from build123d import *

# Parameters (mm, degrees)
SKETCH_1_W          = 85
SKETCH_1_H          = 40
EXTRUDE_1_DEPTH     = 30
SKETCH_2_W          = 60
SKETCH_2_H          = 10
CUT_EXTRUDE_2_DEPTH = 112.467484048
SKETCH_3_R          = 11
CUT_EXTRUDE_3_DEPTH = 99.615414617


with BuildPart() as part:
    # 草图1 → 凸台-拉伸1 (new, symmetric)
    with BuildSketch(Plane.XY):
        with Locations((-42.5, -20)):
            Rectangle(SKETCH_1_W, SKETCH_1_H)
    extrude(amount=EXTRUDE_1_DEPTH, both=True)

    # 草图2 → 切除-拉伸2 (cut, through all)
    with BuildSketch(Plane.XY.offset(30)):
        with Locations((-30, -35)):
            Rectangle(SKETCH_2_W, SKETCH_2_H)
    extrude(amount=-CUT_EXTRUDE_2_DEPTH, mode=Mode.SUBTRACT)

    # 草图3 → 切除-拉伸3 (cut, through all)
    with BuildSketch(Plane(origin=(0, 0, 0), x_dir=(1, 0, 0), z_dir=(0, 1, 0))):
        with Locations(Location((-30, 0, 0), (0, 0, 180))):
            Circle(SKETCH_3_R)
    extrude(amount=-CUT_EXTRUDE_3_DEPTH, mode=Mode.SUBTRACT)


solid = part.part
Source: CAD feature listing. Evaluate the final solid. Frame: model axes, mm. A direction names the side the tool comes from. Give positions to 0.01 mm unless a question says otherwise; leave off trailing zeros. Write each loop counter-clockwise with the first axis right and the second up, starting at its lowest first coordinate (ties: lowest second). Pieces come first, ordered by that corner, then holes. Notation, with made-up numbers: M 13,5.5 L 44,5.5 A5 cw 44,14.5 Z; hole C 36.5,-14 d5. An arc over 180 degrees is marked long. Return JSON: item names as keys, results as strings. Group by question number.
1) Set-up query: faces 1 (the face through (-85, -20, 0)), 2 (the face through (-60, -35, 0)). Return all of +Z, -Z, +X, -X, +Y, -Y with unobstructed straight access to the full face (end or side cutting, diameter ignored); none if empty.
2) Cut plane D-D, the plane z = 17. Output: boundary loops of the cut face in (x, y), then the cut area to 3 significant figures.
3) Draft query along Z for faces 3 (the face through (-40.492, -14.79, 3.304)), 4 (the face through (-73, -40, 0)), 5 (the face through (-43, -15, 30)). Return one class per face: released by +Z, released by -Z, zero draft, split by the parting line, or undercut.
4) Cut plane A-A, the plane z = 0. Output: boundary loops of the cut face in (x, y), then the cut area to 3 significant figures.
5) Ray query, L1, parallel to Z at x = -30.5, y = -26; L2, parallel to Y at x = -57, z = 0; L3, parallel to X at y = -35.5, z = -22. Return the intervals inside material, ascending.
6) First-contact query: pin 1 Ø3 at (y, z) = (-34, -6.5) entering from +X. Flat tip, straight axial feed; report the tip coordinate or a pass-through.
7) Cut plane C-C, the plane y = -14. Output: boundary loops of the cut face in (x, z), then the cut area to 3 significant figures.
8) Cut plane B-B, the plane x = -30. Output: boundary loops of the cut face in (y, z).
Data:
{
 "1": {"face 1": "+Z, -Z, -X, +Y, -Y", "face 2": "+Z, -Z, +X, -Y"},
 "2": {"outline": "M -85,-40 L -60,-40 L -60,-30 L 0,-30 L 0,0 L -85,0 Z", "area": "2,800 mm²"},
 "3": {"face 3": "undercut", "face 4": "zero draft", "face 5": "released by +Z"},
 "4": {"outline": "M -85,-40 L -60,-40 L -60,-30 L -41,-30 L -41,0 L -85,0 Z; M -19,-30 L 0,-30 L 0,0 L -19,0 Z", "area": "2,140 mm²"},
 "5": {"L1": "z = -30 to -10.99, 10.99 to 30", "L2": "y = -30 to 0", "L3": "x = -85 to -60"},
 "6": {"pin 1": "stops at x = -60"},
 "7": {"outline": "M -85,-30 L 0,-30 L 0,30 L -85,30 Z; hole C -30,0 d22", "area": "4,720 mm²"},
 "8": {"outline": "M -30,-30 L 0,-30 L 0,-11 L -30,-11 Z; M -30,11 L 0,11 L 0,30 L -30,30 Z"}
}
